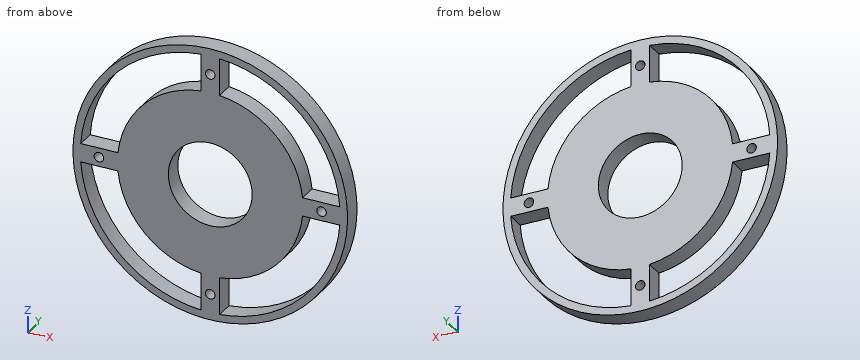
```python
from build123d import *

# Parameters (mm, degrees)
SKETCH1_R           = 46.99
BOSS_EXTRUDE1_DEPTH = 6.35
SKETCH2_R           = 14.351
CUT_EXTRUDE1_DEPTH  = 6.35
CUT_EXTRUDE2_DEPTH  = 6.35
CIRPATTERN1_COUNT   = 4


with BuildPart() as part:
    # Sketch1 → Boss-Extrude1 (new body)
    with BuildSketch(Plane(origin=(0, 0, 0), x_dir=(1, 0, 0), z_dir=(0, 1, 0))):
        with Locations(Location((0, 0, 0), (0, 0, 270))):
            Circle(SKETCH1_R)
    extrude(amount=BOSS_EXTRUDE1_DEPTH)

    # Sketch2 → Cut-Extrude1 (cut)
    with BuildSketch(Plane(origin=(0, 6.35, 0), x_dir=(1, 0, 0), z_dir=(0, 1, 0))):
        with Locations(Location((0, 0, 0), (0, 0, 270))):
            Circle(SKETCH2_R)
    extrude(amount=-CUT_EXTRUDE1_DEPTH, mode=Mode.SUBTRACT)

    # Sketch3 → Cut-Extrude2 (cut)
    with BuildSketch(Plane(origin=(0, 6.35, 0), x_dir=(1, 0, 0), z_dir=(0, 1, 0))):
        with BuildLine():
            ThreePointArc((44.336462139, 3.175), (31.430896424, 31.430896424), (3.175, 44.336462139))
            Line((3.175, 44.336462139), (3.175, 31.590851128))
            ThreePointArc((3.175, 31.590851128), (22.450640303, 22.450640303), (31.590851128, 3.175))
            Line((31.590851128, 3.175), (44.336462139, 3.175))
        make_face()
        with BuildLine():
            Line((-3.175, 31.590851128), (-3.175, 44.336462139))
            ThreePointArc((-3.175, 44.336462139), (-31.430896424, 31.430896424), (-44.336462139, 3.175))
            Line((-44.336462139, 3.175), (-31.590851128, 3.175))
            ThreePointArc((-31.590851128, 3.175), (-22.450640303, 22.450640303), (-3.175, 31.590851128))
        make_face()
        with BuildLine():
            ThreePointArc((3.175, -44.336462139), (31.430896424, -31.430896424), (44.336462139, -3.175))
            Line((44.336462139, -3.175), (31.590851128, -3.175))
            ThreePointArc((31.590851128, -3.175), (22.450640303, -22.450640303), (3.175, -31.590851128))
            Line((3.175, -31.590851128), (3.175, -44.336462139))
        make_face()
        with BuildLine():
            Line((-31.590851128, -3.175), (-44.336462139, -3.175))
            ThreePointArc((-44.336462139, -3.175), (-31.430896424, -31.430896424), (-3.175, -44.336462139))
            Line((-3.175, -44.336462139), (-3.175, -31.590851128))
            ThreePointArc((-3.175, -31.590851128), (-22.450640303, -22.450640303), (-31.590851128, -3.175))
        make_face()
    extrude(amount=-CUT_EXTRUDE2_DEPTH, mode=Mode.SUBTRACT)

    # Sketch4 → 4 Clearance Hole1 (revolve, cut)
    with BuildSketch(Plane(origin=(0, 6.35, -38.1), x_dir=(0, 0, 1), z_dir=(1, 0, 0))):
        Polygon((0, 0), (0, 11.140574487), (1.63195, 10.16), (1.63195, 0), align=None)
    f_4_clearance_hole1 = revolve(axis=Axis((0, 12.7, -38.1), (0, -1, 0)), mode=Mode.SUBTRACT)

    # CirPattern1: 4 Clearance Hole1 ×4 about axis
    cirpattern1_axis = Axis((0, 0, 0), (0, 1, 0))
    for i in range(1, CIRPATTERN1_COUNT):
        add(f_4_clearance_hole1.rotate(cirpattern1_axis, i * 360 / CIRPATTERN1_COUNT), mode=Mode.SUBTRACT)


solid = part.part
```
Verification items for the finished model (mm, model axes). Round coordinates to 2 decimals unless told otherwise and drop trailing zeros. Order: outer loops, then holes, each group sorted by start corner. A loop starts at its lowest first (then second) coordinate and runs counter-clockwise, first axis right, second up. Notation, with made-up numbers: (38.25, -1) - (73.25, -1) arc R34 cw to (73.25, 36) - close; hole circle Ø10 at (-24.75, 72). An arc over 180 degrees is marked (long way). Use CSV: the item, a comma, the result in double quotes.
(1) Gauge pin test, flat ends, axial feed: pin 1 Ø3 at (x, y) = (-35.5, 4) entering from -Z; pin 2 Ø1.9 at (x, y) = (-35.5, 3) entering from +Z; pin 3 Ø2 at (x, z) = (-38.1, 0) entering from +Y; pin 4 Ø3 at (y, z) = (4.5, -41) entering from +X. Record the tip position at first contact, or that the pin passes through.
Entries:
pin 1,"z = -32.44"
pin 2,"z = 31.85"
pin 3,"through"
pin 4,"x = 25.45"
(2) Section check B-B on z = 0. Record the boundary of the cut face in (x, y), and give its area (3 significant figures).
Entries:
outline,"(-46.99, 0) - (-39.73, 0) - (-39.73, 6.35) - (-46.99, 6.35) - close; (-36.47, 0) - (-14.35, 0) - (-14.35, 6.35) - (-36.47, 6.35) - close; (14.35, 0) - (36.47, 0) - (36.47, 6.35) - (14.35, 6.35) - close; (39.73, 0) - (46.99, 0) - (46.99, 6.35) - (39.73, 6.35) - close"
area,"373 mm^2"
(3) Thickness scan on probe 1 along Z at (x, y) = (36, 2.5) (3 decimals); probe 2 along Z at (x, y) = (-19.5, 2.25); probe 3 along Z at (x, y) = (38.1, 2) (3 decimals). Record the ranges inside material, lowest first. Write a range as from..to.
Entries:
probe 1,"-30.2..-26.073, -3.175..3.175, 26.073..30.2"
probe 2,"-42.75..-39.94, -25.06..25.06, 39.94..42.75"
probe 3,"-27.504..-22.895, -3.175..-1.632, 1.632..3.175, 22.895..27.504"
(4) Section check A-A on y = 5. State how many separate pieces and enclosed holes the cut face has, and give its area (3 significant figures).
Entries:
separate pieces,"1"
enclosed holes,"9"
area,"3,540 mm^2"
(5) Section check C-C on x = 0. Record the boundary of the cut face in (y, z).
Entries:
outline,"(0, -46.99) - (6.35, -46.99) - (6.35, -39.73) - (0, -39.73) - close; (0, -36.47) - (6.35, -36.47) - (6.35, -14.35) - (0, -14.35) - close; (0, 14.35) - (6.35, 14.35) - (6.35, 36.47) - (0, 36.47) - close; (0, 39.73) - (6.35, 39.73) - (6.35, 46.99) - (0, 46.99) - close"
(6) Section check D-D on x = -23. Record the boundary of the cut face in (y, z).
Entries:
outline,"(0, -40.98) - (6.35, -40.98) - (6.35, -38.04) - (0, -38.04) - close; (0, -21.89) - (6.35, -21.89) - (6.35, 21.89) - (0, 21.89) - close; (0, 38.04) - (6.35, 38.04) - (6.35, 40.98) - (0, 40.98) - close"
